```python
from build123d import *

# Parameters (mm, degrees)
BOSS_EXTRUDE1_DEPTH      = 20
BOSS_EXTRUDE1_DEPTH_BACK = 41.225
SKETCH1_R                = 7
CUT_EXTRUDE1_START       = -7.225
SKETCH2_R                = 7
SKETCH2_R_2              = 3.96875
CUT_EXTRUDE1_DEPTH       = 36.171941222
SKETCH3_R                = 7
SKETCH3_R_2              = 5
CUT_EXTRUDE2_DEPTH       = 5
SKETCH4_R                = 7
SKETCH4_R_2              = 6.5
CUT_EXTRUDE3_DEPTH       = 41.236799077
CUT_EXTRUDE4_START       = -20
SKETCH5_R                = 6.5
SKETCH5_R_2              = 5
CUT_EXTRUDE4_DEPTH       = 20
CHAMFER1_SIZE            = 0.5
CUT_EXTRUDE5_DEPTH       = 43.237431563


with BuildPart() as part:
    # Sketch1 → Boss-Extrude1 (new, two sides: drawn at the far end of the back side and taken through both)
    with BuildSketch(Plane(origin=(0, 0, 0), x_dir=(0, 0, -1), z_dir=(1, 0, 0)).offset(-BOSS_EXTRUDE1_DEPTH_BACK)):
        Circle(SKETCH1_R)
    extrude(amount=BOSS_EXTRUDE1_DEPTH + BOSS_EXTRUDE1_DEPTH_BACK)

    # Sketch2 → Cut-Extrude1 (cut, through all)
    with BuildSketch(Plane(origin=(0, 0, 0), x_dir=(0, 0, -1), z_dir=(1, 0, 0)).offset(CUT_EXTRUDE1_START)):
        Circle(SKETCH2_R)
        Circle(SKETCH2_R_2, mode=Mode.SUBTRACT)
    extrude(amount=-CUT_EXTRUDE1_DEPTH, mode=Mode.SUBTRACT)

    # Sketch3 → Cut-Extrude2 (cut)
    with BuildSketch(Plane.ZY.offset(7.225)):
        Circle(SKETCH3_R)
        Circle(SKETCH3_R_2, mode=Mode.SUBTRACT)
    extrude(amount=-CUT_EXTRUDE2_DEPTH, mode=Mode.SUBTRACT)

    # Sketch4 → Cut-Extrude3 (cut, through all)
    with BuildSketch(Plane.ZY.offset(2.225)):
        Circle(SKETCH4_R)
        Circle(SKETCH4_R_2, mode=Mode.SUBTRACT)
    extrude(amount=-CUT_EXTRUDE3_DEPTH, mode=Mode.SUBTRACT)

    # Sketch5 → Cut-Extrude4 (cut)
    with BuildSketch(Plane(origin=(20, 0, 0), x_dir=(0, 0, -1), z_dir=(1, 0, 0)).offset(CUT_EXTRUDE4_START)):
        with Locations(Location((0, 0, 0), (0, 0, 180))):
            Circle(SKETCH5_R)
        with Locations(Location((0, 0, 0), (0, 0, 180))):
            Circle(SKETCH5_R_2, mode=Mode.SUBTRACT)
    extrude(amount=CUT_EXTRUDE4_DEPTH, mode=Mode.SUBTRACT)

    # Chamfer1
    chamfer1_edges = [part.edges().sort_by_distance(p)[0] for p in [
        (-7.225, 0, -5),
        (20, 0, -5),
        (-41.225, 0, 3.96875),
    ]]
    chamfer(chamfer1_edges, length=CHAMFER1_SIZE)

    # Sketch6 → Cut-Extrude5 (cut, through all)
    with BuildSketch(Plane(origin=(0, 0, 0), x_dir=(0, 0, -1), z_dir=(1, 0, 0))):
        with BuildLine():
            Line((-6, -2.5), (-6, 2.5))
            ThreePointArc((-6, 2.5), (-6.5, 0), (-6, -2.5))
        make_face()
        with BuildLine():
            Line((6, 2.5), (6, -2.5))
            ThreePointArc((6, -2.5), (6.5, 0), (6, 2.5))
        make_face()
    extrude(amount=-CUT_EXTRUDE5_DEPTH, mode=Mode.SUBTRACT)


solid = part.part
```
The listing builds one solid part. Answer for the finished solid, in the listing's coordinates (mm). A direction names the side the tool comes from. Give positions to 0.01 mm unless a question says otherwise; leave off trailing zeros. Write each loop counter-clockwise with the first axis right and the second up, starting at its lowest first coordinate (ties: lowest second). Pieces come first, ordered by that corner, then holes. Notation, with made-up numbers: (35, 40) - (59, 40) arc R12 ccw to (59, 56) - close; hole circle Ø11 at (40.25, -14.5). An arc over 180 degrees is marked (long way). Use one line per item in the form item = value. Start each with the question number.
1) Find section B-B on z = 0. Determine the outline of the cut face in (x, y) (3 decimals).
2) Flat-ended cylindrical pins translate along their axes: pin 1 Ø4 at (x, z) = (-4.5, 0.5) entering from +Y; pin 2 Ø2 at (x, z) = (9.5, 2.5) entering from +Y; pin 3 Ø6 at (x, z) = (-24.5, 3) entering from -Y. Find the tip coordinate at first contact, or state that the pin passes through.
3) A tool of negligible diameter and unlimited length cuts with its end or side. For faces 1 (the face through (10, 0, -5)), 2 (the face through (-1.1, 6.5, 0.1)), 3 (the face through (-2.225, 4.4, -2.7)), from which of +Z, -Z, +X, -X, +Y, -Y can it reach the whole face along a straight path? Write none if from no direction.
4) Consider line 1 along Z through (x, y) = (-13.5, 0.25); line 2 along X through (y, z) = (5, 2.5) (3 decimals). Determine where each line is inside the solid, lowest interval first. Write a range as from..to.
5) Find section D-D on x = -17. Determine the outline of the cut face in (y, z), plus the area to 3 significant figures.
6) Find section A-A on y = 0. Determine the outline of the cut face in (x, z) (3 decimals).
7) Find section C-C on x = 11. Determine the outline of the cut face in (y, z).
Geometry results:
q1.outline = (-41.225, -3.469) - (-40.725, -3.969) - (-7.225, -3.969) - (-7.225, -4.5) - (-6.725, -5) - (-2.225, -5) - (-2.225, -6.5) - (0, -6.5) - (0, -5) - (19.5, -5) - (20, -4.5) - (20, 4.5) - (19.5, 5) - (0, 5) - (0, 6.5) - (-2.225, 6.5) - (-2.225, 5) - (-6.725, 5) - (-7.225, 4.5) - (-7.225, 3.969) - (-40.725, 3.969) - (-41.225, 3.469) - close
q2.pin_1 = 5
q2.pin_2 = 4.77
q2.pin_3 = -3.97
q3.face_1 = +X
q3.face_2 = +X, -X, +Y
q3.face_3 = -X
q4.line_1 = -3.96..3.96
q4.line_2 = -2.225..0
q5.outline = circle Ø7.94 at (0, 0)
q5.area = 49.5 mm2
q6.outline = (-41.225, -3.469) - (-40.725, -3.969) - (-7.225, -3.969) - (-7.225, -4.5) - (-6.725, -5) - (-2.225, -5) - (-2.225, -6) - (0, -6) - (0, -5) - (19.5, -5) - (20, -4.5) - (20, 4.5) - (19.5, 5) - (0, 5) - (0, 6) - (-2.225, 6) - (-2.225, 5) - (-6.725, 5) - (-7.225, 4.5) - (-7.225, 3.969) - (-40.725, 3.969) - (-41.225, 3.469) - close
q7.outline = circle Ø10 at (0, 0)
